The figure shows three views and two pictorial views of one solid part (mm, origin at its lowest corner). Answer the questions. A direction names the side the tool comes from. Give positions to 0.01 mm unless a question says otherwise; leave off trailing zeros. Order: outer loops, then holes, each group sorted by start corner. A loop starts at its lowest first (then second) coordinate and runs counter-clockwise, first axis right, second up. Notation, with made-up numbers: (61, 30) - (85, 30) arc R9 cw to (85, 39) - close; hole circle Ø4 at (18.25, 88.5). An arc over 180 degrees is marked (long way). Write item = value, one per line.
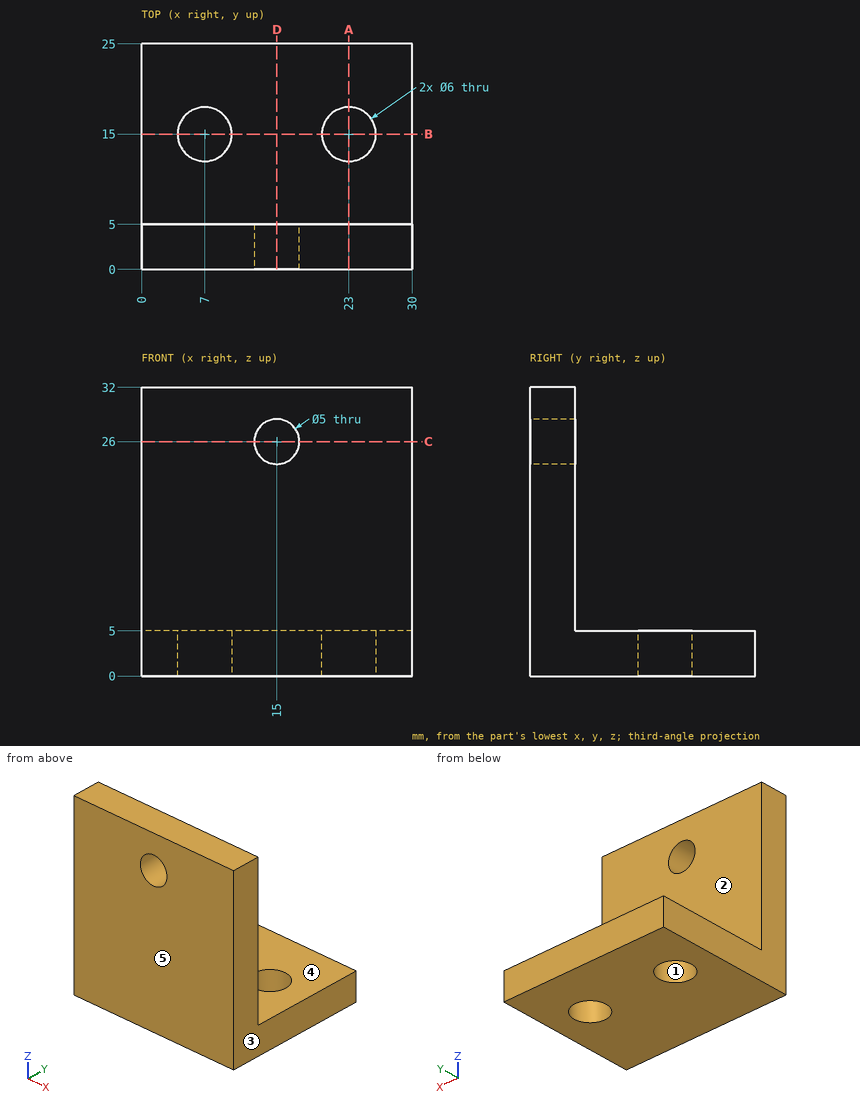
1. Flat-ended cylindrical pins translate along their axes: pin 1 (8 mm diameter, centred on x = 26, z = 25.5, fed in from +Y); pin 2 (2 mm diameter, centred on x = 11, z = 11.5, fed in from -Y); pin 3 (10 mm diameter, centred on x = 15.5, y = 10.5, fed in from +Z). Find the tip coordinate at first contact, or state that the pin passes through.
Recorded:
pin_1 = 5
pin_2 = 0
pin_3 = 5
2. Section D-D (x = 15) is taken. Determine the outline of the cut face in (y, z), and give its area (3 significant figures).
Recorded:
outline = (0, 0) - (25, 0) - (25, 5) - (5, 5) - (5, 23.5) - (0, 23.5) - close; (0, 28.5) - (5, 28.5) - (5, 32) - (0, 32) - close
area = 235 mm^2
3. Section B-B (y = 15) is taken. Determine the outline of the cut face in (x, z), and give its area (3 significant figures).
Recorded:
outline = (0, 0) - (4, 0) - (4, 5) - (0, 5) - close; (10, 0) - (20, 0) - (20, 5) - (10, 5) - close; (26, 0) - (30, 0) - (30, 5) - (26, 5) - close
area = 90.0 mm^2
4. For the marked faces 4 and 5, determine the directions among +Z, -Z, +X, -X, +Y, -Y from which every point of the face is accessible in a straight line to the end or side of a thin tool.
Recorded:
face_4 = +Z, +X, -X, +Y
face_5 = +Z, -Z, +X, -X, -Y
5. Straight lines are drawn through the part: L1, parallel to Y at x = 23, z = 1.85; L2, parallel to Z at x = 11.75, y = 9.75. For each, find the intervals that lie inside material, in ascending order. Write a range as [from, to].
Recorded:
L1 = [0, 12], [18, 25]
L2 = [0, 5]
6. Section A-A (x = 23) is taken. Determine the outline of the cut face in (y, z), and give its area (3 significant figures).
Recorded:
outline = (0, 0) - (12, 0) - (12, 5) - (5, 5) - (5, 32) - (0, 32) - close; (18, 0) - (25, 0) - (25, 5) - (18, 5) - close
area = 230 mm^2
7. Section C-C (z = 26) is taken. Determine the outline of the cut face in (x, y), and give its area (3 significant figures).
Recorded:
outline = (0, 0) - (12.5, 0) - (12.5, 5) - (0, 5) - close; (17.5, 0) - (30, 0) - (30, 5) - (17.5, 5) - close
area = 125 mm^2
8. Determine the mould class of the marked faces 1, 2 and 3 for opening direction X: +X half, -X half, draft (parallel to the pull), parting line (faces both ways), or undercut.
Recorded:
face_1 = undercut
face_2 = draft
face_3 = +X half
